```python
from build123d import *

# Parameters (mm, degrees)
SKETCH1_W           = 109.52
SKETCH1_H           = 90
BOSS_EXTRUDE1_DEPTH = 5
SKETCH2_R           = 1.45
CUT_EXTRUDE1_DEPTH  = 7
SKETCH4_W           = 109.52
SKETCH4_H           = 90
BOSS_EXTRUDE2_DEPTH = 3.5
CHAMFER1_SIZE       = 3.5
CHAMFER1_SIZE2      = 4.171137574
SKETCH5_W           = 100.2
SKETCH5_H           = 79.2
CUT_EXTRUDE3_DEPTH  = 6.5
SKETCH8_R           = 1.45
CUT_EXTRUDE5_DEPTH  = 3


with BuildPart() as part:
    # Sketch1 → Boss-Extrude1 (new body)
    with BuildSketch(Plane.XY):
        with Locations((49.453432203, -35.801949153)):
            Rectangle(SKETCH1_W, SKETCH1_H)
    extrude(amount=BOSS_EXTRUDE1_DEPTH)

    # Sketch2 → Cut-Extrude1 (cut)
    with BuildSketch(Plane(origin=(0, 9.198050847, 0), x_dir=(1, 0, 0), z_dir=(0, 1, 0))):
        with Locations(Location((-2.806567797, -2.5, 0), (0, 0, 270))):
            Circle(SKETCH2_R)
        with Locations(Location((101.713432203, -2.5, 0), (0, 0, 270))):
            Circle(SKETCH2_R)
    extrude(amount=-CUT_EXTRUDE1_DEPTH, mode=Mode.SUBTRACT)

    # Sketch4 → Boss-Extrude2 (add)
    with BuildSketch(Plane(origin=(0, 0, 0), x_dir=(-1, 0, 0), z_dir=(0, 0, -1))):
        with Locations((-49.453432203, -35.801949153)):
            Rectangle(SKETCH4_W, SKETCH4_H)
    extrude(amount=BOSS_EXTRUDE2_DEPTH)

    # Chamfer1
    chamfer1_edges = [part.edges().sort_by_distance(p)[0] for p in [
        (49.453432203, 9.198050847, -3.5),
    ]]
    chamfer1_side = [part.faces().sort_by_distance(p)[0] for p in [
        (49.453432203, 9.198050847, 0.724808812),
    ]]
    chamfer(chamfer1_edges, length=CHAMFER1_SIZE, length2=CHAMFER1_SIZE2, reference=chamfer1_side[0])

    # Sketch5 → Cut-Extrude3 (cut)
    with BuildSketch(Plane(origin=(0, 0, -3.5), x_dir=(-1, 0, 0), z_dir=(0, 0, -1))):
        with Locations((-49.453432203, -35.801949153)):
            Rectangle(SKETCH5_W, SKETCH5_H)
    extrude(amount=-CUT_EXTRUDE3_DEPTH, mode=Mode.SUBTRACT)

    # Sketch8 → Cut-Extrude5 (cut)
    with BuildSketch(Plane(origin=(104.213432203, 0, 0), x_dir=(0, 0, -1), z_dir=(1, 0, 0))):
        with Locations((0.5, -66.551949153)):
            Circle(SKETCH8_R)
    cut_extrude5 = extrude(amount=-CUT_EXTRUDE5_DEPTH, mode=Mode.SUBTRACT)

    # Mirror2: Cut-Extrude5 across plane
    add(cut_extrude5.mirror(Plane.ZY.offset(-49.453432203)), mode=Mode.SUBTRACT)


solid = part.part
```
Build history of the part. All positions in model axes, mm. A direction names the side the tool comes from. Round coordinates to 2 decimals unless told otherwise and drop trailing zeros. Loops run counter-clockwise (first coordinate to the right, second up) from the corner with the lowest first, then second, coordinate; pieces in that order, holes last. Notation, with made-up numbers: M 84.5,79.25 L 108.5,79.25 A24 ccw 108.5,100.25 Z; hole C 62.5,52 d10. An arc over 180 degrees is marked long. Answer as CSV lines item,"result".
1. Cut at B-B on x = 63. Write the cut outline in (y, z).
Resolved:
outline,"M -80.8,-3.5 L -75.4,-3.5 L -75.4,3 L 3.8,3 L 3.8,-3.5 L 5.03,-3.5 L 9.2,0 L 9.2,5 L -80.8,5 Z"
2. Cut at A-A on y = -3.5. Write the cut outline in (x, z).
Resolved:
outline,"M -5.31,-3.5 L -0.65,-3.5 L -0.65,3 L 99.55,3 L 99.55,-3.5 L 104.21,-3.5 L 104.21,5 L -5.31,5 Z"
3. Wall check: probe 1 along X at (y, z) = (5, 2.5); probe 2 along X at (y, z) = (3.5, 2.25); probe 3 along X at (y, z) = (-55.5, 0.5). Give the ranges that are in metal, low to high. Write a range as [from, to].
Resolved:
probe 1,"x = [-5.31, -4.26], [-1.36, 100.26], [103.16, 104.21]"
probe 2,"x = [-5.31, -4.23], [-1.38, -0.65], [99.55, 100.29], [103.14, 104.21]"
probe 3,"x = [-5.31, -0.65], [99.55, 104.21]"
4. Two-plate mould, pull along Z, no slides. Class faces 4 (the cylindrical face through (102.734, -65.114, -0.311)), 5 (the flat face through (50, -76, -3.5)), 6 (the flat face through (49, -35, 5)), 7 (the flat face through (104.213, -36, 1)): released by +Z, released by -Z, zero draft, split by the parting line, or undercut.
Resolved:
face 4,"undercut"
face 5,"released by -Z"
face 6,"released by +Z"
face 7,"zero draft"
5. Flat gauge pins, fed straight in: P1, Ø2, axis at x = 89, z = -1.5, coming from the +Y side; P2, Ø1.7, axis at y = -66.55, z = -0.5, coming from the +X side; P3, Ø3, axis at x = 59, y = -35.5, coming from the -Z side. Where does each tip first touch, or does it go through?
Resolved:
P1,"stops at y = 8.6"
P2,"stops at x = 101.21"
P3,"stops at z = 3"
6. 3-axis set-ups, long thin cutter, end or side, ignore diameter. For faces 1 (the cylindrical face through (103.15, 5.75, 2.31)), 2 (the flat face through (-2.307, -67, 0)), 3 (the flat face through (-0.647, -36, 0)): which of +Z, -Z, +X, -X, +Y, -Y reach the whole face in a straight line?
Resolved:
face 1,"+Y"
face 2,"-X"
face 3,"-Z"
